CAD build for the part. Positions are in the model's coordinates, mm. Face numbers are marked on the shaded views. A direction names the side the tool comes from. Coordinates: 2 decimals unless noted, no trailing zeros. Loops run counter-clockwise (first coordinate to the right, second up) from the corner with the lowest first, then second, coordinate; pieces in that order, holes last.
1) Saw through at D-D, the plane x = 23. Write the cut outline in (y, z), and give its area (3 significant figures).
2) Saw through at C-C, the plane x = 12. Write the cut outline in (y, z), and give its area (3 significant figures).
3) Two-plate mould, pull along Z, no slides. Class the marked faces 1, 2 and 3: +Z half, -Z half, draft (parallel to the pull), parting line (faces both ways), or undercut.
4) Which spindle directions (+Z, -Z, +X, -X, +Y, -Y) get a long thin tool onto all of the face, cutting with end or side? Do the marked faces 4 and 5. Say none if no direction does.
5) Saw through at B-B, the plane y = 18.5. Write the cut outline in (x, z), and give its area (3 significant figures).
6) Saw through at A-A, the plane z = 17.5. Write the cut outline in (x, y), and give its area (3 significant figures).
7) Wall check: line 1 along Y through (x, z) = (23, 2); line 2 along Z through (x, y) = (2.5, 5); line 3 along X through (y, z) = (18, 1). Give the ranges that are in metal, low to high.
8) Pin check, flat tips, straight feed: pin 1 Ø7.5 at (x, y) = (23.5, 4.5) entering from +Z; pin 2 Ø8.5 at (x, z) = (9, 12) entering from -Y; pin 3 Ø0.8 at (x, z) = (10.5, 3.5) entering from -Y. Stop position of each tip, or through.
```python
from build123d import *

# Parameters (mm, degrees)
BOSS_EXTRUDE1_DEPTH = 3
SKETCH2_W           = 15
SKETCH2_H           = 6.5
BOSS_EXTRUDE2_DEPTH = 1.5
BOSS_EXTRUDE3_DEPTH = 4.5
CUT_EXTRUDE1_DEPTH  = 1.5
FILLET1_R           = 0.8
CHAMFER1_SIZE       = 2
CHAMFER2_SIZE       = 2
FILLET2_R           = 0.8
SKETCH5_R           = 2.5
CUT_EXTRUDE2_DEPTH  = 57.384838388
SKETCH6_R           = 2.5
CUT_EXTRUDE3_DEPTH  = 57.384838388


with BuildPart() as part:
    # Sketch1 → Boss-Extrude1 (new body)
    with BuildSketch(Plane.XY):
        Polygon((0, 0), (20, 0), (30, 10), (30, 30), (0, 30), align=None)
    extrude(amount=BOSS_EXTRUDE1_DEPTH)

    # Sketch2 → Boss-Extrude2 (add)
    with BuildSketch(Plane.XY.offset(3)):
        Polygon((30, 10), (15.3, 10), (15.3, 0), (20, 0), align=None)
        with Locations((7.5, 26.75)):
            Rectangle(SKETCH2_W, SKETCH2_H)
    extrude(amount=BOSS_EXTRUDE2_DEPTH)

    # Sketch3 → Boss-Extrude3 (add)
    with BuildSketch(Plane(origin=(0, 30, 0), x_dir=(1, 0, 0), z_dir=(0, 1, 0))):
        Polygon((0, -3), (0, -33), (15, -33), (30, -23), (30, -3), (30, 0), (0, 0), align=None)
    extrude(amount=BOSS_EXTRUDE3_DEPTH)

    # Sketch4 → Cut-Extrude1 (cut)
    with BuildSketch(Plane.XZ.offset(-30)):
        Polygon((15, 23), (30, 23), (30, 3), (15, 3), (15, 4.5), align=None)
    extrude(amount=-CUT_EXTRUDE1_DEPTH, mode=Mode.SUBTRACT)

    # Fillet1
    fillet1_edges = [part.edges().sort_by_distance(p)[0] for p in [
        (15, 23.5, 3.75),
        (7.5, 23.5, 4.5),
        (15, 26.75, 4.5),
        (15.3, 5, 4.5),
        (15.3, 10, 3.75),
        (22.65, 10, 4.5),
        (15, 30, 13.75),
        (22.5, 30, 23),
        (15, 30.75, 23),
    ]]
    fillet(fillet1_edges, radius=FILLET1_R)

    # Chamfer1
    chamfer1_edges = [part.edges().sort_by_distance(p)[0] for p in [
        (15, 34.5, 0),
    ]]
    chamfer(chamfer1_edges, length=CHAMFER1_SIZE)

    # Chamfer2
    # the kernel refuses this chamfer: 2 mm, written as the material it takes off along each edge
    with BuildSketch(Plane(origin=(30, 37.643365976, 0), x_dir=(-0.9996219169112968, 0, -0.02749587661058639), z_dir=(0, -1, 0))) as chamfer2_piece_1:
        Polygon((CHAMFER2_SIZE * 0.999621916911, -CHAMFER2_SIZE * 0.0274958766106), (-CHAMFER2_SIZE * 0.0274958766106, -CHAMFER2_SIZE * 0.999621916911), (0, 0), align=None)
    extrude(amount=32.786731952, mode=Mode.SUBTRACT)
    with BuildSketch(Plane(origin=(16.36309104, -3.63690896, 0), x_dir=(-0.7068394360706732, 0.7068394360706737, -0.027495876610586376), z_dir=(0.7071067811865478, 0.7071067811865474, 0))) as chamfer2_piece_2:
        Polygon((CHAMFER2_SIZE * 0.999621916911, CHAMFER2_SIZE * 0.0274958766106), (-CHAMFER2_SIZE * 0.0274958766106, CHAMFER2_SIZE * 0.999621916911), (0, 0), align=None)
    extrude(amount=24.428867576, mode=Mode.SUBTRACT)
    with BuildSketch(Plane(origin=(-5.143365976, 0, 0), x_dir=(0, 0.9996219169112968, -0.027495876610586372), z_dir=(1, 0, 0))) as chamfer2_piece_3:
        Polygon((CHAMFER2_SIZE * 0.999621916911, CHAMFER2_SIZE * 0.0274958766106), (-CHAMFER2_SIZE * 0.0274958766106, CHAMFER2_SIZE * 0.999621916911), (0, 0), align=None)
    extrude(amount=30.286731952, mode=Mode.SUBTRACT)
    with BuildSketch(Plane(origin=(0, 37.643365976, 0), x_dir=(-0.027495876610586372, 0, 0.9996219169112968), z_dir=(0, -1, 0))) as chamfer2_piece_4:
        Polygon((CHAMFER2_SIZE * 0.999621916911, -CHAMFER2_SIZE * 0.0274958766106), (-CHAMFER2_SIZE * 0.0274958766106, -CHAMFER2_SIZE * 0.999621916911), (0, 0), align=None)
    extrude(amount=42.786731952, mode=Mode.SUBTRACT)
    with BuildSketch(Plane(origin=(0, 34.5, 38.143365976), x_dir=(-0.0274958766105864, -0.9996219169112968, 0), z_dir=(0, 0, -1))) as chamfer2_piece_5:
        Polygon((CHAMFER2_SIZE * 0.999621916911, -CHAMFER2_SIZE * 0.0274958766106), (-CHAMFER2_SIZE * 0.0274958766106, -CHAMFER2_SIZE * 0.999621916911), (0, 0), align=None)
    extrude(amount=41.286731952, mode=Mode.SUBTRACT)
    with BuildSketch(Plane(origin=(30, 34.5, -3.143365976), x_dir=(-0.9996219169112968, 0.027495876610585647, 0), z_dir=(0, 0, 1))) as chamfer2_piece_6:
        Polygon((CHAMFER2_SIZE * 0.999621916911, CHAMFER2_SIZE * 0.0274958766106), (-CHAMFER2_SIZE * 0.0274958766106, CHAMFER2_SIZE * 0.999621916911), (0, 0), align=None)
    extrude(amount=31.286731952, mode=Mode.SUBTRACT)
    with BuildSketch(Plane(origin=(10.720460826, 34.5, 35.853026116), x_dir=(-0.5544904734617357, 0.027495876610585605, -0.8317357101926042), z_dir=(0.8320502943378439, 0, -0.5547001962252288))) as chamfer2_piece_7:
        Polygon((CHAMFER2_SIZE * 0.999621916911, -CHAMFER2_SIZE * 0.0274958766106), (-CHAMFER2_SIZE * 0.0274958766106, -CHAMFER2_SIZE * 0.999621916911), (0, 0), align=None)
    extrude(amount=28.314488329, mode=Mode.SUBTRACT)
    with BuildSketch(Plane(origin=(-5.143365976, 34.5, 33), x_dir=(0, 0.027495876610585647, -0.9996219169112968), z_dir=(1, 0, 0))) as chamfer2_piece_8:
        Polygon((CHAMFER2_SIZE * 0.999621916911, -CHAMFER2_SIZE * 0.0274958766106), (-CHAMFER2_SIZE * 0.0274958766106, -CHAMFER2_SIZE * 0.999621916911), (0, 0), align=None)
    extrude(amount=25.286731952, mode=Mode.SUBTRACT)

    # Fillet2
    fillet2_edges = [part.edges().sort_by_distance(p)[0] for p in [
        (22.5, 31.5, 3),
    ]]
    fillet(fillet2_edges, radius=FILLET2_R)

    # Sketch5 → Cut-Extrude2 (cut, through all)
    with BuildSketch(Plane(origin=(0, 0, 0), x_dir=(-1, 0, 0), z_dir=(0, 0, -1))):
        with Locations((-23, 18.5)):
            Circle(SKETCH5_R)
    extrude(amount=-CUT_EXTRUDE2_DEPTH, mode=Mode.SUBTRACT)

    # Sketch6 → Cut-Extrude3 (cut, through all)
    with BuildSketch(Plane(origin=(0, 34.5, 0), x_dir=(1, 0, 0), z_dir=(0, 1, 0))):
        with Locations(Location((23, -16, 0), (0, 0, 180))):
            Circle(SKETCH6_R)
    extrude(amount=-CUT_EXTRUDE3_DEPTH, mode=Mode.SUBTRACT)


solid = part.part
```
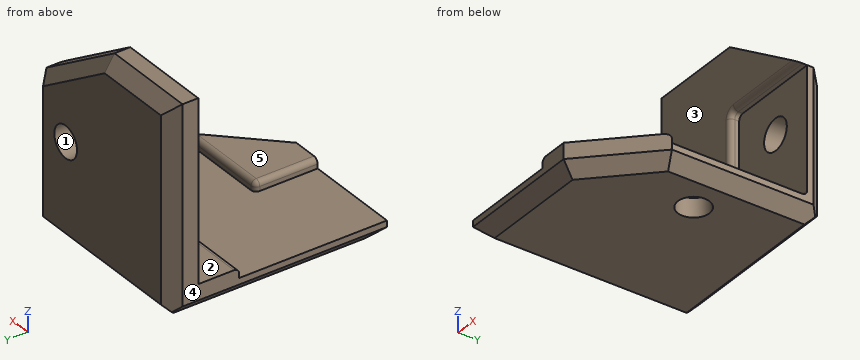
Data:
1. outline: (3, 2) - (5.83, 0) - (16, 0) - (16, 3) - (10, 3) - (10, 3.7) arc R0.8 ccw to (9.2, 4.5) - (3, 4.5) - close; (21, 0) - (32.5, 0) - (34.5, 2) - (34.5, 13.5) - (31.5, 13.5) - (31.5, 3.8) arc R0.8 cw to (30.7, 3) - (21, 3) - close; (30, 23.8) arc R0.8 ccw to (30.8, 23) - (31.5, 23) - (31.5, 18.5) - (34.5, 18.5) - (34.5, 25.26) - (32.5, 27.67) - (30, 27.67) - close
1. area: 149 mm2
2. outline: (0, 2) - (2, 0) - (32.5, 0) - (34.5, 2) - (34.5, 31) - (32.5, 33) - (30, 33) - (30, 4.5) - (24.3, 4.5) arc R0.8 ccw to (23.5, 3.7) - (23.5, 3) - (0, 3) - close
2. area: 242 mm2
3. face 1: undercut
3. face 2: +Z half
3. face 3: draft
4. face 4: +Z, -Z, -X, +Y, -Y
4. face 5: +Z, +X, -X, -Y
5. outline: (0, 2) - (2, 0) - (20.5, 0) - (20.5, 3) - (0, 3) - close; (25.5, 0) - (28, 0) - (30, 2) - (30, 3) - (25.5, 3) - close
5. area: 71.0 mm2
6. outline: (0, 30) - (14.2, 30) arc R0.8 ccw to (15, 30.8) - (15, 31.5) - (21, 31.5) - (21, 34.5) - (2, 34.5) - (0, 32.5) - close; (25, 31.5) - (30, 31.5) - (30, 32.5) - (28, 34.5) - (25, 34.5) - close
6. area: 96.4 mm2
7. line 1: y = 3 to 16, 21 to 34.5
7. line 2: z = 0 to 3
7. line 3: x = 1 to 20.55, 25.45 to 29
8. pin 1: stops at z = 4.5
8. pin 2: stops at y = 30
8. pin 3: stops at y = 23.5
